Source: CAD feature listing. Evaluate the final solid. Frame: model axes, mm. A direction names the side the tool comes from. Round coordinates to 2 decimals unless told otherwise and drop trailing zeros. Order: outer loops, then holes, each group sorted by start corner. A loop starts at its lowest first (then second) coordinate and runs counter-clockwise, first axis right, second up. Notation, with made-up numbers: (89, -7.75) - (113, -7.75) arc R21 ccw to (113, 9.25) - close; hole circle Ø7 at (-8, -39). An arc over 180 degrees is marked (long way). Return JSON: item names as keys, results as strings. Group by question number.
1) Section A-A, the plane z = 0.6. Return loops of the section in (x, y).
2) Section C-C, the plane y = 1.25. Return loops of the section in (x, z), plus the area to 3 significant figures.
3) Contact query for flat-ended pins moving along their axis: P1, Ø2.5, axis at y = 2.5, z = 1.5, coming from the -X side; P2, Ø1.5, axis at x = 3.5, z = 1.5, coming from the -Y side. Output: stop coordinate, or through.
4) Ray query, line 1 (Y direction, x = -11, z = 2.8); line 2 (X direction, y = 7.75, z = 2.2). Return the intervals inside material, ascending. Write a range as from..to.
5) Access query for faces 1 (the flat face through (5, 12, 2)), 2 (the flat face through (0, 5, 2)), 3 (the flat face through (-10, 5, 2)). Directions: +Z, -Z, +X, -X, +Y, -Y. A direction counts if a zero-diameter tool reaches every point of the face in a straight line with its end or side. Return the directions, or none.
6) Section B-B, the plane x = -11.25. Return loops of the section in (y, z).
```python
from build123d import *

# Parameters (mm, degrees)
SKETCH1_W           = 10
SKETCH1_H           = 10
BOSS_EXTRUDE1_DEPTH = 5


with BuildPart() as part:
    # Sketch1 → Boss-Extrude1 (new body)
    with BuildSketch(Plane.XY):
        Polygon((-10, 10), (0, 10), (5, 10), (5, 15), (-15, 15), (-15, 10), align=None)
        with Locations((-5, 5)):
            Rectangle(SKETCH1_W, SKETCH1_H)
    extrude(amount=BOSS_EXTRUDE1_DEPTH)


solid = part.part
```
Geometry check:
{
 "1": {"outline": "(-15, 10) - (-10, 10) - (-10, 0) - (0, 0) - (0, 10) - (5, 10) - (5, 15) - (-15, 15) - close"},
 "2": {"outline": "(-10, 0) - (0, 0) - (0, 5) - (-10, 5) - close", "area": "50.0 mm2"},
 "3": {"P1": "x = -10", "P2": "y = 10"},
 "4": {"line 1": "10..15", "line 2": "-10..0"},
 "5": {"face 1": "+Z, -Z, +X, +Y, -Y", "face 2": "+Z, -Z, +X, -Y", "face 3": "+Z, -Z, -X, -Y"},
 "6": {"outline": "(10, 0) - (15, 0) - (15, 5) - (10, 5) - close"}
}
